from build123d import *

# Parameters (mm, degrees)
F0_W     = 101.6
F0_H     = 76.2
F1_DEPTH = 63.5
F3_DEPTH = 101.6
F4_W     = 50.8
F4_H     = 38.1
F5_DEPTH = 25.4


with BuildPart() as f1:
    # F0 (on Front) → F1 (new body)
    with BuildSketch(Plane.XZ):
        with Locations((-4.7626945901, -22.2168454429)):
            Rectangle(F0_W, F0_H)
    extrude(amount=F1_DEPTH)

    # F2 (on face) → F3 (cut)
    with BuildSketch(Plane.YZ.offset(46.0373054099)):
        with BuildLine():
            ThreePointArc((-63.5, -34.9168454429), (-27.5789755157, -20.0378699272), (-12.7, 15.8831545571))
            Line((-12.7, 15.8831545571), (-63.5, 15.8831545571))
            Line((-63.5, 15.8831545571), (-63.5, -34.9168454429))
        make_face()
    extrude(amount=-F3_DEPTH, mode=Mode.SUBTRACT)

    # F4 (on face) → F5 (cut)
    with BuildSketch(Plane(origin=(0, 0, 0), x_dir=(-1, 0, 0), z_dir=(0, 1, 0))):
        with Locations((5.135083878, -3.1668454429)):
            Rectangle(F4_W, F4_H)
    extrude(amount=-F5_DEPTH, mode=Mode.SUBTRACT)


solid = f1.part
Could you check a few things on this model? Use its own coordinates, in mm. A direction names the side the tool comes from. Round coordinates to 2 decimals unless told otherwise and drop trailing zeros. Order: outer loops, then holes, each group sorted by start corner. A loop starts at its lowest first (then second) coordinate and runs counter-clockwise, first axis right, second up. Notation, with made-up numbers: M 51.25,65 L 109.25,65 A21 cw 109.25,86 Z; hole C 17,84.25 d1. An arc over 180 degrees is marked long. One line per item, written item: value.
(1) Imagine slicing it at C-C (x = 1.5). Write out the boundary of the cut face in (y, z), and give its area (3 significant figures).
Ans:
outline: M -63.5,-60.32 L 0,-60.32 L 0,-22.22 L -25.4,-22.22 L -25.4,-17.72 A50.8 cw -63.5,-34.92 Z
area: 2,140 mm^2
(2) If we mould it in two halves opening along X, with no side actions, what happens to faces 1 (the flat face through (-55.563, -24, -31)), 2 (the flat face through (20.265, -10, -8)), 3 (the flat face through (33, -6, 15.883))? For each: released by +X, released by -X, zero draft, split by the parting line, or undercut.
Ans:
face 1: released by -X
face 2: undercut
face 3: zero draft
(3) I need wall thicknesses on line 1 along X through (y, z) = (-5, -14); line 2 along Z through (x, y) = (-7, -12.5); line 3 along Z through (x, y) = (37, -34). Which ranges of each line are inside material? Lowest first, please. Write a range as from..to.
Ans:
line 1: x = -55.56..-30.54, 20.26..46.04
line 2: z = -60.32..-22.22
line 3: z = -60.32..-25.47
(4) Which directions (+Z, -Z, +X, -X, +Y, -Y) give clear straight access to the entire face, cutting with the end or side of a thin tool? Please do faces 4 (the flat face through (-5, -63.5, -47)), 5 (the flat face through (-5, -25.4, -20)).
Ans:
face 4: +Z, -Z, +X, -X, -Y
face 5: +Z, +Y
(5) Imagine slicing it at A-A (z = 10). Write out the boundary of the cut face in (x, y).
Ans:
outline: M -55.56,-13.04 L -30.54,-13.04 L -30.54,0 L -55.56,0 Z; M 20.26,-13.04 L 46.04,-13.04 L 46.04,0 L 20.26,0 Z
(6) Imagine slicing it at B-B (y = -5.5). Write out the boundary of the cut face in (x, z), and give its area (3 significant figures).
Ans:
outline: M -55.56,-60.32 L 46.04,-60.32 L 46.04,15.88 L 20.26,15.88 L 20.26,-22.22 L -30.54,-22.22 L -30.54,15.88 L -55.56,15.88 Z
area: 5,810 mm^2
(7) I'm going to push flat-ended pins straight in: P1, Ø6, axis at x = -11, y = -14.5, coming from the +Z side; P2, Ø12, axis at y = -24.5, z = -4, coming from the +X side; P3, Ø2, axis at x = -2.5, z = -19.5, coming from the +Y side; P4, Ø10, axis at x = 23, y = -30.5, coming from the +Z side. Where does each tip first touch, or does it pass through?
Ans:
P1: stops at z = -22.22
P2: passes through
P3: stops at y = -25.4
P4: stops at z = -17.83
(8) Imagine slicing it at D-D (z = -10). Write out the boundary of the cut face in (x, y).
Ans:
outline: M -55.56,-19.79 L -30.54,-19.79 L -30.54,0 L -55.56,0 Z; M 20.26,-19.79 L 46.04,-19.79 L 46.04,0 L 20.26,0 Z
